from build123d import *

# Parameters (mm, degrees)
Y_KSEKLIK_EKSTR_ZYON1_DEPTH = 30
IZIM2_R                     = 25
Y_KSEKLIK_EKSTR_ZYON2_DEPTH = 60
IZIM3_R                     = 12.5
KES_EKSTR_ZYON1_DEPTH       = 158.638827704
L_O_ALTMA2_COUNT            = 2
L_O_ALTMA2_PITCH            = 190
L_O_ALTMA2_COUNT_DIR2       = 2
L_O_ALTMA2_PITCH_DIR2       = 90


with BuildPart() as part:
    # Çizim1 → Yükseklik-Ekstrüzyon1 (new body)
    with BuildSketch(Plane(origin=(0, 0, 0), x_dir=(1, 0, 0), z_dir=(0, 1, 0))):
        with BuildLine():
            Line((-115, 75), (115, 75))
            ThreePointArc((115, 75), (122.071067812, 72.071067812), (125, 65))
            Line((125, 65), (125, -65))
            ThreePointArc((125, -65), (122.071067812, -72.071067812), (115, -75))
            Line((115, -75), (-115, -75))
            ThreePointArc((-115, -75), (-122.071067812, -72.071067812), (-125, -65))
            Line((-125, -65), (-125, 65))
            ThreePointArc((-125, 65), (-122.071067812, 72.071067812), (-115, 75))
        make_face()
    extrude(amount=-Y_KSEKLIK_EKSTR_ZYON1_DEPTH)

    # Çizim2 → Yükseklik-Ekstrüzyon2 (add)
    with BuildSketch(Plane(origin=(0, 0, 0), x_dir=(1, 0, 0), z_dir=(0, 1, 0))):
        with Locations(Location((0, 25, 0), (0, 0, 90))):
            Circle(IZIM2_R)
    extrude(amount=Y_KSEKLIK_EKSTR_ZYON2_DEPTH)

    # Çizim3 → Kes-Ekstrüzyon1 (cut, through all)
    with BuildSketch(Plane(origin=(0, 0, 0), x_dir=(1, 0, 0), z_dir=(0, 1, 0))):
        with Locations(Location((-95, 45, 0), (0, 0, 270))):
            Circle(IZIM3_R)
    kes_ekstr_zyon1 = extrude(amount=-KES_EKSTR_ZYON1_DEPTH, mode=Mode.SUBTRACT)

    # LÇoğaltma2: Kes-Ekstr_zyon1 2 × 2
    with Locations(*[(i * L_O_ALTMA2_PITCH, 0, j * L_O_ALTMA2_PITCH_DIR2) for i in range(L_O_ALTMA2_COUNT) for j in range(L_O_ALTMA2_COUNT_DIR2) if (i, j) != (0, 0)]):
        add(kes_ekstr_zyon1, mode=Mode.SUBTRACT)


solid = part.part
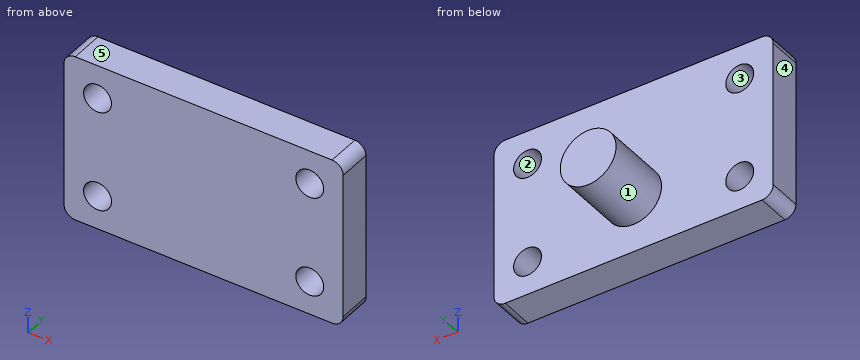
The listing builds one solid part. Answer for the finished solid, in the listing's coordinates (mm). Face numbers are marked on the shaded views. A direction names the side the tool comes from. Give positions to 0.01 mm unless a question says otherwise; leave off trailing zeros. Write each loop counter-clockwise with the first axis right and the second up, starting at its lowest first coordinate (ties: lowest second). Pieces come first, ordered by that corner, then holes.
1) Section C-C (z = -25) is taken. Write down the section's boundary in (x, y), and give its area (3 significant figures).
2) Section D-D (x = 0) is taken. Write down the section's boundary in (y, z), and give its area (3 significant figures).
3) Section B-B (z = -45) is taken. Write down the section's boundary in (x, y).
4) A tool of negligible diameter and unlimited length cuts with its end or side. For the marked faces 1 and 2, from which of +Z, -Z, +X, -X, +Y, -Y can it reach the whole face along a straight path? Write none if from no direction.
5) Find the intervals of material crossed by L1, parallel to X at y = -9.5, z = -45; L2, parallel to Y at x = -7.5, z = 23.5; L3, parallel to X at y = -24.5, z = 51, in increasing order.
6) For a pull along Z with two mould halves and no side action, classify the marked faces 3, 4 and 5 as pulls with the +Z half, pulls with the -Z half, needs draft (parallel to the pull), parting line crosses it, or undercut.
7) Given P1, Ø8, axis at x = 26, y = 28, coming from the -Z side; P2, Ø8, axis at x = 25.5, z = -48.5, coming from the +Y side; P3, Ø8, axis at x = -98, y = 3, coming from the -Z side, each flat-ended and moving along its own axis, determine where each tip first touches the part or whether it passes through.
8) Section A-A (x = -95) is taken. Write down the section's boundary in (y, z).
Response:
1. outline: (-125, -30) - (125, -30) - (125, 0) - (25, 0) - (25, 60) - (-25, 60) - (-25, 0) - (-125, 0) - close
1. area: 10,500 mm2
2. outline: (-30, -75) - (0, -75) - (0, -50) - (60, -50) - (60, 0) - (0, 0) - (0, 75) - (-30, 75) - close
2. area: 7,500 mm2
3. outline: (-125, -30) - (-107.5, -30) - (-107.5, 0) - (-125, 0) - close; (-82.5, -30) - (82.5, -30) - (82.5, 0) - (15, 0) - (15, 60) - (-15, 60) - (-15, 0) - (-82.5, 0) - close; (107.5, -30) - (125, -30) - (125, 0) - (107.5, 0) - close
4. face 1: +Y
4. face 2: +Y, -Y
5. L1: x = -125 to -107.5, -82.5 to 82.5, 107.5 to 125
5. L2: y = -30 to 0
5. L3: x = -125 to -105.97, -84.03 to 84.03, 105.97 to 125
6. face 3: undercut
6. face 4: needs draft
6. face 5: pulls with the +Z half
7. P1: stops at z = -36.87
7. P2: stops at y = 0
7. P3: stops at z = -75
8. outline: (-30, -75) - (0, -75) - (0, -57.5) - (-30, -57.5) - close; (-30, -32.5) - (0, -32.5) - (0, 32.5) - (-30, 32.5) - close; (-30, 57.5) - (0, 57.5) - (0, 75) - (-30, 75) - close
